Part model, mm, in its own coordinate system. Face numbers are marked on the shaded views. A direction names the side the tool comes from. Give positions to 0.01 mm unless a question says otherwise; leave off trailing zeros. Order: outer loops, then holes, each group sorted by start corner. A loop starts at its lowest first (then second) coordinate and runs counter-clockwise, first axis right, second up. Notation, with made-up numbers: (75, -14) - (105, -14) arc R30 ccw to (105, 10) - close; hole circle Ø7 at (69.25, 1.5). An arc over 180 degrees is marked (long way). Use one line per item in the form item = value. Start each with the question number.
1. Pull direction Z, two halves, no side cores. Call the marked faces 5, 6 and 7: +Z half, -Z half, draft (parallel to the pull), parting line (faces both ways), or undercut.
2. Band-saw the part on B-B, the plane y = 14. List the corners of the cut face in (x, z), plus the area to 3 significant figures.
3. Drill centre lines: line 1 (Y direction, x = 25, z = 3.5); line 2 (X direction, y = 2.75, z = 1); line 3 (X direction, y = 10.5, z = 3.5). Where is each one in solid material? Low to high.
4. Tool access for the marked faces 1, 2, 3 and 4: list every direction of +Z, -Z, +X, -X, +Y, -Y with a clear straight run to the whole face (end or side of a thin tool).
5. Pin check, flat tips, straight feed: P1, Ø1.8, axis at x = 25, y = 0, coming from the -Z side; P2, Ø10.5, axis at x = -24.5, z = 12.5, coming from the +Y side; P3, Ø3, axis at x = 11.5, z = 6, coming from the +Y side; P4, Ø3.5, axis at x = 20, z = 14.5, coming from the -Y side. Stop position of each tip, or through.
6. Band-saw the part on C-C, the plane x = 0. List the corners of the cut face in (y, z), plus the area to 3 significant figures.
7. Band-saw the part on A-A, the plane z = 23.5. List the corners of the cut face in (x, y).
8. Band-saw the part on D-D, the plane z = 8.75. List the corners of the cut face in (x, y).
from build123d import *

# Parameters (mm, degrees)
BOSS_EXTRU_1_DEPTH      = 25
ESQUISSE2_R             = 2.375
BOSS_EXTRU_2_DEPTH      = 5
ESQUISSE3_R             = 1.5
BOSS_EXTRU_3_DEPTH      = 7.5
ESQUISSE4_R             = 1.5
BOSS_EXTRU_4_DEPTH      = 7.5
ESQUISSE5_W             = 11.114887109
ESQUISSE5_H             = 10.09418398
ENL_V_MAT_EXTRU_1_DEPTH = 10


with BuildPart() as part:
    # Esquisse1 → Boss.-Extru.1 (new body)
    with BuildSketch(Plane.XY):
        with BuildLine():
            Line((-17.435595774, 1.5), (-21.44761059, 1.5))
            ThreePointArc((-21.44761059, 1.5), (0.750457302, 21.486898656), (21.5, 0))
            Line((21.5, 0), (17.5, 0))
            ThreePointArc((17.5, 0), (0.750690999, 17.48389153), (-17.435595774, 1.5))
        make_face()
    extrude(amount=BOSS_EXTRU_1_DEPTH)

    # Esquisse2 → Boss.-Extru.2 (add)
    with BuildSketch(Plane.XZ.offset(-1.5)):
        with BuildLine():
            Line((-17.435595774, 7.5), (-24.935595774, 7.5))
            ThreePointArc((-24.935595774, 7.5), (-29.935595774, 12.5), (-24.935595774, 17.5))
            Line((-24.935595774, 17.5), (-17.435595774, 17.5))
            Line((-17.435595774, 17.5), (-17.435595774, 7.5))
        make_face()
        with Locations((-24.935595774, 12.5)):
            Circle(ESQUISSE2_R, mode=Mode.SUBTRACT)
    extrude(amount=-BOSS_EXTRU_2_DEPTH)

    # Esquisse3 → Boss.-Extru.3 (add)
    with BuildSketch(Plane.XY.offset(25)):
        with BuildLine():
            Line((17.5, -3.5), (25, -3.5))
            ThreePointArc((25, -3.5), (28.5, 0), (25, 3.5))
            Line((25, 3.5), (17.5, 3.5))
            Line((17.5, 3.5), (17.5, -3.5))
        make_face()
        with Locations((25, 0)):
            Circle(ESQUISSE3_R, mode=Mode.SUBTRACT)
    extrude(amount=-BOSS_EXTRU_3_DEPTH)

    # Esquisse4 → Boss.-Extru.4 (add)
    with BuildSketch(Plane(origin=(0, 0, 0), x_dir=(-1, 0, 0), z_dir=(0, 0, -1))):
        with BuildLine():
            Line((-17.5, -3.5), (-25, -3.5))
            ThreePointArc((-25, -3.5), (-28.5, 0), (-25, 3.5))
            Line((-25, 3.5), (-17.5, 3.5))
            Line((-17.5, 3.5), (-17.5, -3.5))
        make_face()
        with Locations((-25, 0)):
            Circle(ESQUISSE4_R, mode=Mode.SUBTRACT)
    extrude(amount=-BOSS_EXTRU_4_DEPTH)

    # Esquisse5 → Enlèv. mat.-Extru.1 (cut)
    with BuildSketch(Plane(origin=(0, 0, 17.5), x_dir=(-1, 0, 0), z_dir=(0, 0, -1))):
        with Locations((-19.442556445, -1.54709199)):
            Rectangle(ESQUISSE5_W, ESQUISSE5_H)
    extrude(amount=ENL_V_MAT_EXTRU_1_DEPTH, mode=Mode.SUBTRACT)


solid = part.part
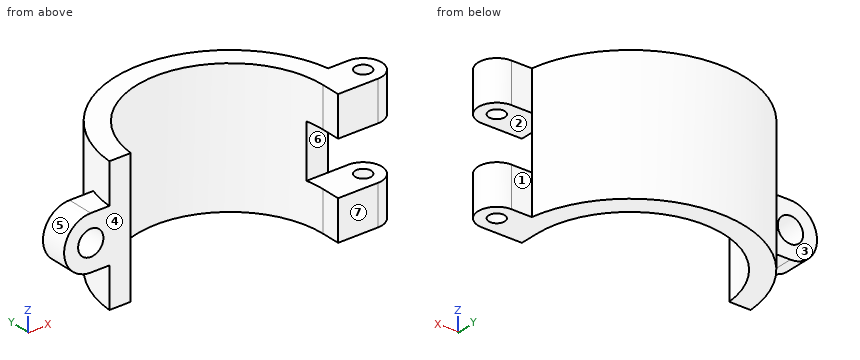
From the geometry:
q1.face_5 = parting line
q1.face_6 = undercut
q1.face_7 = draft
q2.outline = (-16.32, 0) - (-10.5, 0) - (-10.5, 25) - (-16.32, 25) - close; (10.5, 0) - (16.32, 0) - (16.32, 25) - (10.5, 25) - close
q2.area = 291 mm²
q3.line_1 = -3.5 to -1.5, 1.5 to 3.5
q3.line_2 = -21.32 to -17.28, 17.28 to 27.17
q3.line_3 = -18.76 to -14, 14 to 18.76
q4.face_1 = +Z, -Z, +X, +Y
q4.face_2 = +X, -Y
q4.face_3 = +Z, -Z, -X, +Y
q4.face_4 = +Z, -Z, -X, -Y
q5.P1 = through
q5.P2 = 9.58
q5.P3 = 19.03
q5.P4 = 3.5
q6.outline = (17.5, 0) - (21.5, 0) - (21.5, 25) - (17.5, 25) - close
q6.area = 100 mm²
q7.outline = (-21.45, 1.5) - (-17.44, 1.5) arc R17.5 cw to (17.5, 0) - (17.5, -3.5) - (25, -3.5) arc R3.5 ccw to (25, 3.5) - (21.21, 3.5) arc R21.5 ccw to start; hole circle Ø3 at (25, 0)
q8.outline = (-28.24, 1.5) - (-17.44, 1.5) arc R17.5 cw to (17.15, 3.5) - (21.21, 3.5) arc R21.5 ccw to (-20.49, 6.5) - (-28.24, 6.5) - close
